from build123d import *

# Parameters (mm, degrees)
F0_R     = 12.5
F1_DEPTH = 25
F2_W     = 11
F2_H     = 23.5
F4_W     = 147.382453084
F4_H     = 22.0085635483
F5_DEPTH = 55.001
F6_W     = 11
F6_H     = 11
F11_W    = 11
F11_H    = 22


with BuildPart() as f1:
    # F0 (on Top) → F1 (new body)
    with BuildSketch(Plane.XY):
        with BuildLine():
            ThreePointArc((0, 17.5), (5.1256313292, 5.1256313292), (17.5, 0))
            Line((17.5, 0), (110, 0))
            ThreePointArc((110, 0), (113.5355339059, 1.4644660941), (115, 5))
            Line((115, 5), (115, 50))
            ThreePointArc((115, 50), (113.5355339059, 53.5355339059), (110, 55))
            Line((110, 55), (5, 55))
            ThreePointArc((5, 55), (1.4644660941, 53.5355339059), (0, 50))
            Line((0, 50), (0, 17.5))
        make_face()
        with Locations((17.5, 17.5)):
            Circle(F0_R, mode=Mode.SUBTRACT)
    extrude(amount=F1_DEPTH)

    # F2 (on face) → F3 (revolve, cut)
    with BuildSketch(Plane.XY.offset(25)):
        with Locations((40.5, 15.75)):
            Rectangle(F2_W, F2_H)
        with Locations((56.5, 15.75)):
            Rectangle(F2_W, F2_H)
    revolve(axis=Axis((40.5, 27.5, 25), (1, 0, 0)), mode=Mode.SUBTRACT)

    # F4 (on face) → F5 (cut, through all)
    with BuildSketch(Plane.XZ):
        with Locations((73.691226542, 29.0042817742)):
            Rectangle(F4_W, F4_H)
    extrude(amount=-F5_DEPTH, mode=Mode.SUBTRACT)

    # F6 (on face) → F7 (revolve, cut)
    with BuildSketch(Plane.XY.offset(18)):
        with Locations((72.5, 9.5)):
            Rectangle(F6_W, F6_H)
    revolve(axis=Axis((72.5, 15, 18), (1, 0, 0)), mode=Mode.SUBTRACT)

    # F6 (on face) → F8 (revolve, cut)
    with BuildSketch(Plane.XY.offset(18)):
        with Locations((88.5, 21.5)):
            Rectangle(F6_W, F6_H)
    revolve(axis=Axis((88.5, 27, 18), (1, 0, 0)), mode=Mode.SUBTRACT)

    # F6 (on face) → F9 (revolve, cut)
    with BuildSketch(Plane.XY.offset(18)):
        with Locations((72.5, 44.5)):
            Rectangle(F6_W, F6_H)
    revolve(axis=Axis((72.5, 39, 18), (1, 0, 0)), mode=Mode.SUBTRACT)

    # F11 (on offset) → F12 (revolve, cut)
    with BuildSketch(Plane.XY.offset(25)):
        with Locations((104.5, 16)):
            Rectangle(F11_W, F11_H)
    revolve(axis=Axis((104.5, 27, 25), (1, 0, 0)), mode=Mode.SUBTRACT)


solid = f1.part
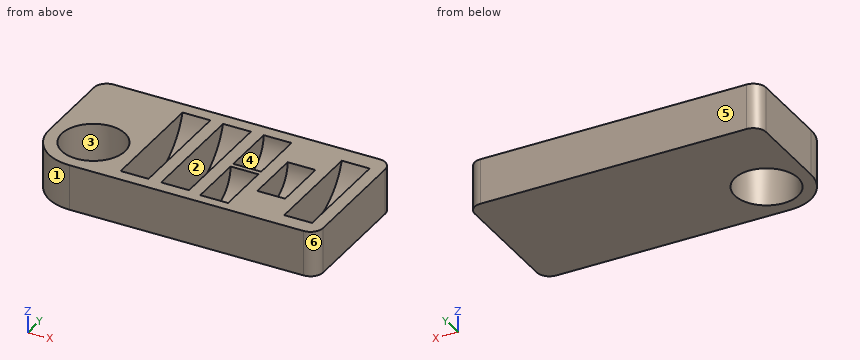
Could you check a few things on this model? Use its own coordinates, in mm. Face numbers are marked on the shaded views. A direction names the side the tool comes from. Give positions to 0.01 mm unless a question says otherwise; leave off trailing zeros. Order: outer loops, then holes, each group sorted by start corner. A loop starts at its lowest first (then second) coordinate and runs counter-clockwise, first axis right, second up. Notation, with made-up numbers: (8, 42.25) - (52, 42.25) arc R24 ccw to (52, 59.25) - close; hole circle Ø6 at (-28, 66). An arc over 180 degrees is marked (long way). Return JSON: item names as keys, results as strings. Group by question number.
Q1. Will these pins go through, and if not, where does the flat tip stop? pin 1 Ø5 at (x, y) = (38.5, 31) entering from +Z; pin 2 Ø2 at (x, y) = (53, 23.5) entering from +Z.
Q2. Suppose I cut it at C-C, the plane z = 14.5. State how many separate pieces and enclosed holes the cut face has, and give its area (3 significant figures).
Q3. Suppose I cut it at D-D, the plane y = 9. Please give me the cut outline in (x, z).
Q4. Suppose I cut it at B-B, the plane x = 85.5. Please give me the cut outline in (y, z).
Q5. Thinking about a two-plate mould opening in X: for the marked faces 3, 4, 5 and 6, which applies, pulls with the +X half, pulls with the -X half, needs draft (parallel to the pull), parting line crosses it, or undercut?
Q6. Which directions (+Z, -Z, +X, -X, +Y, -Y) give clear straight access to the entire face, cutting with the end or side of a thin tool? Please do the marked faces 1 and 2.
Q7. Please list where these lines run through material, in increasing order: line 1 along X through (y, z) = (17.5, 11); line 2 along X through (y, z) = (17.5, 5); line 3 along X through (y, z) = (17.5, 6). Write a range as [from, to].
Q8. Suppose I cut it at A-A, the plane x = 21. Please give me the cut outline in (y, z), and give its area (3 significant figures).
Resolved:
{
 "1": {"pin 1": "stops at z = 2.28", "pin 2": "stops at z = 2.04"},
 "2": {"separate pieces": "1", "enclosed holes": "7", "area": "3,710 mm2"},
 "3": {"outline": "(2.2, 0) - (8.33, 0) - (8.33, 18) - (2.2, 18) - close; (26.67, 0) - (115, 0) - (115, 18) - (110, 18) - (110, 12.35) - (99, 12.35) - (99, 18) - (78, 18) - (78, 8.78) - (67, 8.78) - (67, 18) - (62, 18) - (62, 10.51) - (51, 10.51) - (51, 18) - (46, 18) - (46, 10.51) - (35, 10.51) - (35, 18) - (26.67, 18) - close"},
 "4": {"outline": "(0, 0) - (55, 0) - (55, 18) - (38, 18) arc R11 cw to (16, 18) - (0, 18) - close"},
 "5": {"face 3": "undercut", "face 4": "undercut", "face 5": "needs draft", "face 6": "pulls with the +X half"},
 "6": {"face 1": "+Z, -Z, -X, -Y", "face 2": "+Z"},
 "7": {"line 1": "x = [0, 5], [30, 35], [46, 51], [62, 67], [78, 99], [110, 115]", "line 2": "x = [0, 5], [30, 35], [46, 51], [62, 115]", "line 3": "x = [0, 5], [30, 35], [46, 51], [62, 99], [110, 115]"},
 "8": {"outline": "(0, 0) - (5.5, 0) - (5.5, 18) - (0, 18) - close; (29.5, 0) - (55, 0) - (55, 18) - (29.5, 18) - close", "area": "558 mm2"}
}
